Answer from the drawing. Dimensions are ordinates in mm from the lowest x, y and z of the part. A direction names the side the tool comes from. Give positions to 0.01 mm unless a question says otherwise; leave off trailing zeros. Write each loop counter-clockwise with the first axis right and the second up, starting at its lowest first coordinate (ties: lowest second). Pieces come first, ordered by that corner, then holes.
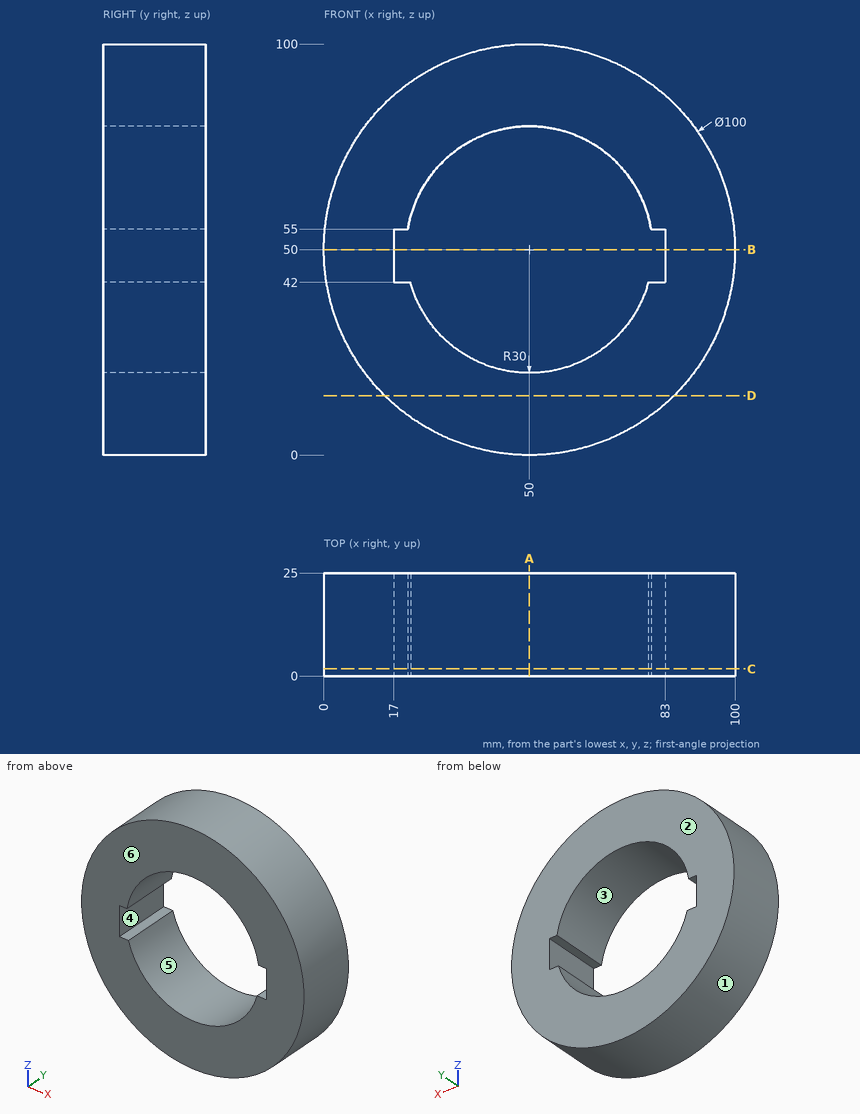
Item 1: A cutting plane is placed at B-B, the plane z = 50. Give the vertices of the cut face in (x, y), plus the area to 3 significant figures.
Conclusion:
outline: (0, 0) - (17, 0) - (17, 25) - (0, 25) - close; (83, 0) - (100, 0) - (100, 25) - (83, 25) - close
area: 850 mm2
Item 2: Consider probe 1 along Z at (x, y) = (51, 8.5); probe 2 along Z at (x, y) = (61.5, 1.5); probe 3 along X at (y, z) = (2.75, 50). Determine where each line is inside the solid, lowest interval first.
Conclusion:
probe 1: z = 0.01 to 20.02, 79.98 to 99.99
probe 2: z = 1.34 to 22.29, 77.71 to 98.66
probe 3: x = 0 to 17, 83 to 100
Item 3: A cutting plane is placed at C-C, the plane y = 1.75. Give the vertices of the cut face in (x, z), plus the area to 3 significant figures.
Conclusion:
outline: circle Ø100 at (50, 50); hole (17, 42) - (21.09, 42) arc R30 ccw to (78.91, 42) - (83, 42) - (83, 55) - (79.58, 55) arc R30 ccw to (20.42, 55) - (17, 55) - close
area: 4,940 mm2
Item 4: Determine the mould class of the marked faces 1, 2, 3 and 4 for opening direction Z: pulls with the +Z half, pulls with the -Z half, needs draft (parallel to the pull), parting line crosses it, or undercut.
Conclusion:
face 1: parting line crosses it
face 2: needs draft
face 3: undercut
face 4: undercut
Item 5: Which of the six approach directions +Z, -Z, +X, -X, +Y, -Y give full straight-line access (tool end or side, diameter ignored) to the marked faces 5 and 6?
Conclusion:
face 5: +Y, -Y
face 6: +Z, -Z, +X, -X, -Y
Item 6: A cutting plane is placed at D-D, the plane z = 14.5. Give the vertices of the cut face in (x, y), plus the area to 3 significant figures.
Conclusion:
outline: (14.79, 0) - (85.21, 0) - (85.21, 25) - (14.79, 25) - close
area: 1,760 mm2
Item 7: Each of these flat-tipped pins is pushed along its axis until it touches: P1, Ø12, axis at x = 16.5, y = 6.5, coming from the +Z side; P2, Ø1, axis at y = 17.5, z = 16.5, coming from the +X side; P3, Ø1, axis at x = 81, y = 14, coming from the -Z side. Where does it stop, or does it pass through?
Conclusion:
P1: stops at z = 91.76
P2: stops at x = 87.56
P3: stops at z = 10.38
Item 8: A cutting plane is placed at A-A, the plane x = 50. Give the vertices of the cut face in (y, z), plus the area to 3 significant figures.
Conclusion:
outline: (0, 0) - (25, 0) - (25, 20) - (0, 20) - close; (0, 80) - (25, 80) - (25, 100) - (0, 100) - close
area: 1,000 mm2
